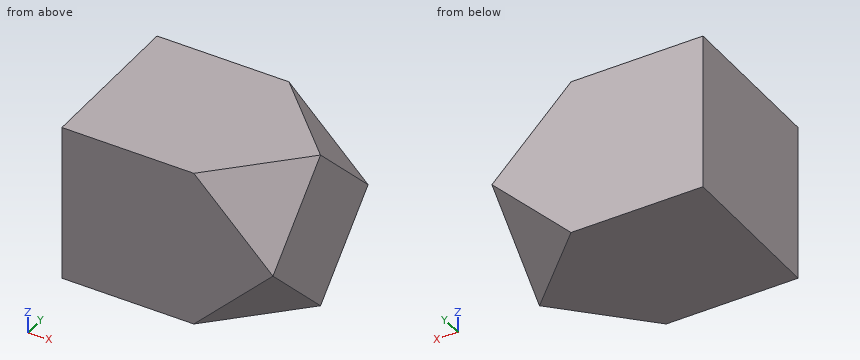
from build123d import *

# Parameters (mm, degrees)
F0_W      = 12.5
F0_H      = 15
F1_DEPTH  = 15
F7_DEPTH  = 25
F10_DEPTH = 43.5
F14_DEPTH = 25
F17_DEPTH = 25


with BuildPart() as f1:
    # F0 (on Front) → F1 (new body)
    with BuildSketch(Plane.XZ):
        with Locations((6.25, 7.5)):
            Rectangle(F0_W, F0_H)
        Polygon((20, 15), (12.5, 15), (20, 7.5), align=None)
        Polygon((20, 7.5), (12.5, 0), (20, 0), align=None)
        Polygon((20, 7.5), (12.5, 15), (12.5, 0), align=None)
    extrude(amount=F1_DEPTH)

    # F6 (on 3pt) → F7 (cut)
    with BuildSketch(Plane(origin=(9.1666666667, 9.1666666667, 9.1666666667), x_dir=(0.8164965809, -0.4082482905, -0.4082482905), z_dir=(-0.5773502692, -0.5773502692, -0.5773502692))):
        Polygon((4.0824829046, 10.6066017178), (13.2680694401, 5.3033008589), (13.2680694401, 15.9099025767), align=None)
    extrude(amount=-F7_DEPTH, mode=Mode.SUBTRACT)

    # F9 (on 3pt) → F10 (cut)
    with BuildSketch(Plane(origin=(4.1666666667, 4.1666666667, -4.1666666667), x_dir=(-0.8164965809, 0.4082482905, -0.4082482905), z_dir=(0.5773502692, 0.5773502692, -0.5773502692))):
        Polygon((-19.391793797, 5.3033008589), (-19.391793797, -5.3033008589), (-10.2062072616, 0), align=None)
    extrude(amount=F10_DEPTH, mode=Mode.SUBTRACT)

    # F13 (on 3pt) → F14 (cut)
    with BuildSketch(Plane(origin=(9.1666666667, -9.1666666667, -9.1666666667), x_dir=(-0.4082482905, -0.8164965809, 0.4082482905), z_dir=(-0.5773502692, 0.5773502692, 0.5773502692))):
        Polygon((-2.0412414523, 14.1421356237), (7.1443450831, 8.8388347648), (7.1443450831, 19.4454364826), align=None)
    extrude(amount=-F14_DEPTH, mode=Mode.SUBTRACT)

    # F16 (on 3pt) → F17 (cut)
    with BuildSketch(Plane(origin=(14.1666666667, -14.1666666667, 14.1666666667), x_dir=(-0.8164965809, -0.4082482905, 0.4082482905), z_dir=(-0.5773502692, 0.5773502692, -0.5773502692))):
        Polygon((2.0412414523, 0), (-7.1443450831, 5.3033008589), (-7.1443450831, -5.3033008589), align=None)
    extrude(amount=-F17_DEPTH, mode=Mode.SUBTRACT)


solid = f1.part
Verification items for the finished model (mm, model axes). Round coordinates to 2 decimals unless told otherwise and drop trailing zeros. Loops run counter-clockwise (first coordinate to the right, second up) from the corner with the lowest first, then second, coordinate; pieces in that order, holes last. Notation, with made-up numbers: (60.5, -10.75) - (82.5, -10.75) arc R24 cw to (82.5, -0.75) - close; hole circle Ø9 at (-17, -12.75). An arc over 180 degrees is marked (long way). Write item = value, one per line.
Q1. Sectioned sample at B-B on z = 5. Record the boundary of the cut face in (x, y).
Here are the results:
outline = (0, -15) - (17.5, -15) - (20, -12.5) - (20, -2.5) - (17.5, 0) - (0, 0) - close
Q2. Material ranges on L1, parallel to X at y = -11.5, z = 3.5; L2, parallel to Z at x = 19.25, y = -9; L3, parallel to X at y = -1.75, z = 12.5, recorded low to high.
Here are the results:
L1 = 0 to 19.5
L2 = 0.75 to 14.25
L3 = 0 to 16.75
Q3. Sectioned sample at A-A on x = 14.25. Record the boundary of the cut face in (y, z), plus the area to 3 significant figures.
Here are the results:
outline = (-15, 1.75) - (-13.25, 0) - (-1.75, 0) - (0, 1.75) - (0, 13.25) - (-1.75, 15) - (-13.25, 15) - (-15, 13.25) - close
area = 219 mm^2
Q4. Depth check by flat-ended pin: pin 1 (6 mm diameter, centred on y = -12.5, z = 11.5, fed in from +X). Enter the tip coordinate at first touch or a pass-through.
Here are the results:
pin_1 = 20
Q5. Sectioned sample at C-C on y = -2.5. Record the boundary of the cut face in (x, z), plus the area to 3 significant figures.
Here are the results:
outline = (0, 0) - (15, 0) - (20, 5) - (20, 10) - (15, 15) - (0, 15) - close
area = 275 mm^2
Q6. Sectioned sample at D-D on x = 18. Record the boundary of the cut face in (y, z).
Here are the results:
outline = (-15, 5.5) - (-9.5, 0) - (-5.5, 0) - (0, 5.5) - (0, 9.5) - (-5.5, 15) - (-9.5, 15) - (-15, 9.5) - close
